Build history of the part. All positions in model axes, mm. A direction names the side the tool comes from. Give positions to 0.01 mm unless a question says otherwise; leave off trailing zeros. Loops run counter-clockwise (first coordinate to the right, second up) from the corner with the lowest first, then second, coordinate; pieces in that order, holes last. Notation, with made-up numbers: (47.25, 46) - (74.25, 46) arc R16 ccw to (74.25, 55) - close; hole circle Ø3 at (3, -11.5). An arc over 180 degrees is marked (long way). Return JSON: item names as keys, results as strings. Group by question number.
1) Slice it at B-B (z = 22.5). List the corners of the cut face in (x, y).
2) Slice it at C-C (z = 6.5). List the corners of the cut face in (x, y).
3) 3-axis set-ups, long thin cutter, end or side, ignore diameter. For faces 1 (the face through (-60.2, -19.87, 27.88)), 2 (the face through (-20, 1, -1.2)): which of +Z, -Z, +X, -X, +Y, -Y reach the whole face in a straight line?
4) Drill centre lines: probe 1 along Y at (x, z) = (11.5, 21); probe 2 along X at (y, z) = (14, 11.5); probe 3 along Y at (x, z) = (-61, 52). Where is each one in solid material? Low to high. Write a range as from..to.
5) Slice it at A-A (x = 2.5). List the corners of the cut face in (y, z), and give its area (4 significant figures).
6) Mould opens along X. For faces 3 (the face through (19.475, -10.995, 52.217)), 4 (the face through (20.127, 22.458, 26.507)), 5 (the face through (-62.272, 0, 27)), 6 (the face through (-20, -20.472, 27)) say: released by +X, released by -X, zero draft, split by the parting line, or undercut.
7) Drop flat-ended pins along their axis: pin 1 (5 mm diameter, centred on x = -14.5, y = 13.5, fed in from +Z); pin 2 (3 mm diameter, centred on y = 13.03, z = 52, fed in from +X); pin 3 (2.5 mm diameter, centred on y = -11.97, z = 52, fed in from -X). Give the stop position or say it passes through.
8) Slice it at D-D (x = -23.5). List the corners of the cut face in (y, z), and give its area (3 significant figures).
Autodesk Inventor part; units mm, degrees
ref_plane "YZ Plane" through (0, 0, 0) normal (1, 0, 0) x (0, 1, 0)
ref_plane "XZ Plane" through (0, 0, 0) normal (0, 1, 0) x (-1, 0, 0)
ref_plane "XY Plane" through (0, 0, 0) normal (0, 0, 1) x (1, 0, 0)
sketch "Sketch1" plane through (0, 0, 0) normal (0, 0, 1) x (1, 0, 0)
  line L0 (-60.7718, 21.5285) -> (19.2282, 21.5285)
  line L1 (19.2282, 21.5285) -> (19.2282, -20.4715)
  line L2 (19.2282, -20.4715) -> (-60.7718, -20.4715)
  line L3 (-60.7718, -20.4715) -> (-60.7718, 21.5285)
  line L4 (-62.2718, 23.0285) -> (20.7282, 23.0285)
  line L5 (20.7282, 23.0285) -> (20.7282, -21.9715)
  line L6 (20.7282, -21.9715) -> (-62.2718, -21.9715)
  line L7 (-62.2718, -21.9715) -> (-62.2718, 23.0285)
  point P0 (0, 0)
  dimension "d0" = 80
  dimension "d1" = 42
  dimension "d2" = 1.5
  dimension "d3" = 1.5
  dimension "d4" = 1.5
  dimension "d5" = 1.5
extrude "Extrusion1" add sketch "Sketch1" along normal blind 55
sketch "Sketch2" plane through (0, 0, 0) normal (0, 0, -1) x (-1, 0, 0)
  line L0 (-20.7282, 23.0285) -> (62.2718, 23.0285)
  line L1 (62.2718, -21.9715) -> (-20.7282, -21.9715)
  line L2 (-20.7282, 23.0285) -> (62.2718, 23.0285)
  line L3 (62.2718, 23.0285) -> (62.2718, -21.9715)
  line L4 (62.2718, -21.9715) -> (-20.7282, -21.9715)
  line L5 (-20.7282, -21.9715) -> (-20.7282, 23.0285)
  point P0 (0, 0)
  point P1 (62.2718, 23.0285)
extrude "Extrusion2" add sketch "Sketch2" along normal blind 1.2
sketch "Sketch3" plane through (-62.2718, -21.9715, 55) normal (-1, 0, 0) x (0, 0, 1)
  line L0 (-40, 27) -> (-44, 27)
  line L1 (-44, 27) -> (-44, 18)
  line L2 (-44, 18) -> (-40, 18)
  line L3 (-40, 18) -> (-40, 27)
  line L4 (-55, 1.5) -> (-55, 43.5)
  line L5 (-55, 1.5) -> (0, 1.5)
  line L6 (-55, 43.5) -> (0, 43.5)
  point P0 (-55, 21.9715)
  dimension "d10" = 11
  dimension "d11" = 15
  dimension "d12" = 9
  dimension "d13" = 16.5
  dimension "d14" = 16.5
extrude "Extrusion3" cut sketch "Sketch3" against normal blind 2
chamfer "Chamfer1" distance 1.5 angle 45 4 edges at (-62.2718, 0.5285, 15) (-62.2718, 0.5285, 11) (-62.2718, 5.0285, 13) (-62.2718, -3.9715, 13)
sketch "Sketch4" plane through (-62.2718, -21.9715, 55) normal (0, -1, 0) x (1, 0, 0)
  line L0 (58.5, -52) -> (78.5, -52)
  line L1 (78.5, -52) -> (78.5, -37)
  line L2 (78.5, -37) -> (58.5, -37)
  line L3 (58.5, -37) -> (58.5, -52)
  line L4 (81.5, -55) -> (1.5, -55)
  line L5 (81.5, -55) -> (81.5, 0)
  point P0 (62.2718, -55)
  dimension "d20" = 3
  dimension "d21" = 3
  dimension "d22" = 20
  dimension "d23" = 15
extrude "Extrusion4" cut sketch "Sketch4" against normal blind 2
fillet "Fillet1" radius 2 8 edges at (19.2282, 21.5285, 27.5) (20.7282, 23.0285, 26.9) (19.2282, -20.4715, 27.5) (20.7282, -21.9715, 26.9) (-60.7718, -20.4715, 27.5) (-62.2718, -21.9715, 26.9) (-60.7718, 21.5285, 27.5) (-62.2718, 23.0285, 26.9)
sketch "Sketch5" plane through (-62.2718, -19.9715, -1.2) normal (-1, 0, 0) x (0, 0, 1)
  line L0 (56.2, 41) -> (56.2, 0)
  line L1 (0, -2) -> (56.2, -2)
  line L2 (56.2, 43) -> (0, 43)
  point P0 (1.2, 19.9715)
  point P1 (53.2, 8)
  point P2 (53.2, 33)
  dimension "d27" = 3
  dimension "d28" = 3
  dimension "d29" = 10
  dimension "d30" = 10
hole "Hole1" at (-62.2718, -11.9715, 52) at (-62.2718, 13.0285, 52) direction (1, 0, 0) diameter 2 depth 10 tip angle 179 countersink diameter 4 countersink angle 90
sketch "Sketch6" plane through (20.7282, -19.9715, -1.2) normal (1, 0, 0) x (0, 0, -1)
  circle A0 centre (-53.2, 33) radius 1
  circle A1 centre (-53.2, 8) radius 1
  point P0 (-1.2, 19.9715)
hole "Hole2" at (20.7282, 13.0285, 52) at (20.7282, -11.9715, 52) direction (-1, 0, 0) diameter 2 depth 10 tip angle 179 countersink diameter 4 countersink angle 90
properties part number "battery case"
Results:
{
 "1": {"outline": "(-62.27, -19.97) arc R2 ccw to (-60.27, -21.97) - (18.73, -21.97) arc R2 ccw to (20.73, -19.97) - (20.73, 21.03) arc R2 ccw to (18.73, 23.03) - (-60.27, 23.03) arc R2 ccw to (-62.27, 21.03) - close; hole (-60.77, -18.47) arc R2 ccw to (-58.77, -20.47) - (17.23, -20.47) arc R2 ccw to (19.23, -18.47) - (19.23, 19.53) arc R2 ccw to (17.23, 21.53) - (-58.77, 21.53) arc R2 ccw to (-60.77, 19.53) - close"},
 "2": {"outline": "(-62.27, -19.97) arc R2 ccw to (-60.27, -21.97) - (-3.77, -21.97) - (-3.77, -20.47) - (-58.77, -20.47) arc R2 cw to (-60.77, -18.47) - (-60.77, 19.53) arc R2 cw to (-58.77, 21.53) - (17.23, 21.53) arc R2 cw to (19.23, 19.53) - (19.23, -18.47) arc R2 cw to (17.23, -20.47) - (16.23, -20.47) - (16.23, -21.97) - (18.73, -21.97) arc R2 ccw to (20.73, -19.97) - (20.73, 21.03) arc R2 ccw to (18.73, 23.03) - (-60.27, 23.03) arc R2 ccw to (-62.27, 21.03) - close"},
 "3": {"face 1": "+Z", "face 2": "-Z, +X, -X, +Y, -Y"},
 "4": {"probe 1": "-21.97..-20.47, 21.53..23.03", "probe 2": "-62.27..-60.77, 19.23..20.73", "probe 3": "-21.83..-12.97, -10.97..12.03, 14.03..22.89"},
 "5": {"outline": "(-21.97, -1.2) - (23.03, -1.2) - (23.03, 55) - (21.53, 55) - (21.53, 0) - (-20.47, 0) - (-20.47, 3) - (-21.97, 3) - close; (-21.97, 18) - (-20.47, 18) - (-20.47, 55) - (-21.97, 55) - close", "area": "196.5 mm2"},
 "6": {"face 3": "zero draft", "face 4": "released by +X", "face 5": "released by -X", "face 6": "undercut"},
 "7": {"pin 1": "z = 0", "pin 2": "x = 20.23", "pin 3": "x = -61.52"},
 "8": {"outline": "(-21.97, -1.2) - (23.03, -1.2) - (23.03, 55) - (21.53, 55) - (21.53, 0) - (-20.47, 0) - (-20.47, 55) - (-21.97, 55) - close", "area": "219 mm2"}
}
